from build123d import *

# Parameters (mm, degrees)
F1_DEPTH = 63.5
F2_DEPTH = 25.4
F3_DEPTH = 9.525
F5_R     = 5.08


with BuildPart() as f1:
    # F0 (on Front) → F1 (new body, symmetric)
    with BuildSketch(Plane.XZ):
        Polygon((41.275, -9.525), (41.275, 9.525), (22.225, 9.525), (-41.275, 9.525), (-41.275, -9.525), align=None)
    extrude(amount=F1_DEPTH, both=True)

    # F0 (on Front) → F2 (join, symmetric)
    with BuildSketch(Plane.XZ):
        with BuildLine():
            Line((22.225, 9.525), (41.275, 9.525))
            Line((41.275, 9.525), (41.275, 27.0002))
            ThreePointArc((41.275, 27.0002), (45.92468, 38.22552), (57.15, 42.8752))
            Line((57.15, 42.8752), (77.695822, 42.8752))
            Line((77.695822, 42.8752), (77.695822, 61.9252))
            Line((77.695822, 61.9252), (57.15, 61.9252))
            add(Edge.make_bspline(
                [(56.136897, 61.910503), (56.476094, 61.9168), (56.813813, 61.921701), (57.15, 61.9252)],
                knots=[110.545926, 110.545926, 110.545926, 110.545926, 111.504536, 111.504536, 111.504536, 111.504536], degree=3))
            ThreePointArc((56.136897, 61.910503), (32.09867, 51.335082), (22.225, 27.0002))
            Line((22.225, 27.0002), (22.225, 9.525))
        make_face()
        Polygon((77.695822, 61.9252), (77.695822, 42.8752), (77.695822, 38.1), (128.495822, 38.1), (128.495822, 66.675), (77.695822, 66.675), align=None)
    extrude(amount=F2_DEPTH, both=True)

    # F0 (on Front) → F3 (join, symmetric)
    with BuildSketch(Plane.XZ):
        with BuildLine():
            Line((-41.275, 9.525), (22.225, 9.525))
            Line((22.225, 9.525), (22.225, 27.0002))
            ThreePointArc((22.225, 27.0002), (32.09867, 51.335082), (56.136897, 61.910503))
            add(Edge.make_bspline(
                [(-41.275, 9.525), (-41.7684, 41.876246), (17.020968, 61.184278), (56.136897, 61.910503)],
                knots=[0, 0, 0, 0, 110.545926, 110.545926, 110.545926, 110.545926], degree=3))
        make_face()
    extrude(amount=F3_DEPTH, both=True)

    # F0 (on Front) → F4 (revolve)
    with BuildSketch(Plane.XZ):
        Polygon((77.695822, 61.9252), (77.695822, 42.8752), (77.695822, 38.1), (128.495822, 38.1), (128.495822, 66.675), (77.695822, 66.675), align=None)
    revolve(axis=Axis((128.495822, 0, 52.3875), (0, 0, 1)))

    # F5
    f5_edges = [f1.edges().sort_by_distance(p)[0] for p in [
        (41.275, 63.5, 0),
        (0, 63.5, 9.525),
        (-41.275, 63.5, 0),
        (0, 63.5, -9.525),
        (41.275, -63.5, 0),
        (0, -63.5, 9.525),
        (-41.275, -63.5, 0),
        (0, -63.5, -9.525),
    ]]
    fillet(f5_edges, radius=F5_R)


solid = f1.part
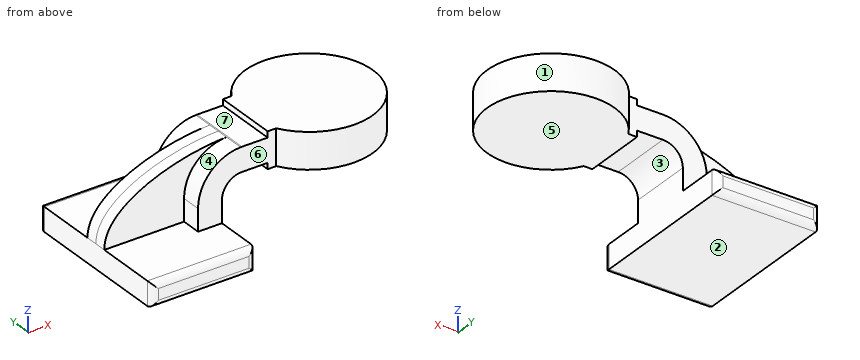
Design review of the part built by this model. Coordinates are the model's own, in mm. Face numbers are marked on the shaded views. A direction names the side the tool comes from. Round coordinates to 2 decimals unless told otherwise and drop trailing zeros. Write each loop counter-clockwise with the first axis right and the second up, starting at its lowest first coordinate (ties: lowest second). Pieces come first, ordered by that corner, then holes. Notation, with made-up numbers: (18.25, 0) -> (39.25, 0) arc R28 cw to (39.25, 23) -> close; hole circle Ø11 at (77.25, 37). An arc over 180 degrees is marked (long way). One line per question, with ' | ' between items.
(1) Take a section at A-A, the plane y = -46. State the section outline as (x, z) points (3 decimals).
Result sheet:
outline: (-41.275, -9.525) -> (41.275, -9.525) -> (41.275, 9.525) -> (-41.275, 9.525) -> close; (106.94, 38.1) -> (150.051, 38.1) -> (150.051, 66.675) -> (106.94, 66.675) -> close
(2) Machinability: for the marked faces 5, 6 and 7, which of the approach directions +Z, -Z, +X, -X, +Y, -Y give a long, thin tool a straight path to every point of the face, cutting with its end or side? Answer none if there is none.
Result sheet:
face 5: -Z, +X, +Y, -Y | face 6: +Z, -X, -Y | face 7: +Z, -X, +Y, -Y
(3) Draft analysis for pull direction X (two halves, no side actions). For the marked faces 1, 2, 3 and 4, state which applies: released by +X, released by -X, zero draft, split by the parting line, or undercut.
Result sheet:
face 1: split by the parting line | face 2: zero draft | face 3: undercut | face 4: released by -X
(4) Take a section at B-B, the plane x = 139. State the section outline as (y, z) points (3 decimals), and give its area (3 significant figures).
Result sheet:
outline: (-49.702, 38.1) -> (49.702, 38.1) -> (49.702, 66.675) -> (-49.702, 66.675) -> close | area: 2,840 mm2
(5) Insertion check: P1, Ø1.4, axis at y = 3.5, z = 39.5, coming from the -X side; P2, Ø5, axis at y = 14.5, z = 18, coming from the -X side (3 decimals); P3, Ø8, axis at y = -19, z = 47, coming from the -X side. Each pin has a flat end and moves straight along its axis. Give the tip position at first contact, or say it passes through.
Result sheet:
P1: x = -22.92 | P2: x = 22.225 | P3: x = 26.11
(6) Wall thickness on line 1 (Y direction, x = 29, z = 15); line 2 (Z direction, x = 91, y = 0.5) (3 decimals); line 3 (X direction, y = -56, z = 1.5) (3 decimals): over which ranges is each line inside the solid? List them lowest first. Write a range as [from, to].
Result sheet:
line 1: [-25.4, 25.4] | line 2: [38.1, 66.675] | line 3: [-41.275, 41.275]
